from build123d import *

# Parameters (mm, degrees)
SKETCH3_R                                         = 22
BOSS_EXTRUDE1_DEPTH                               = 1.5
BOSS_EXTRUDE2_DEPTH                               = 12.5
SKETCH5_R                                         = 24.5
SKETCH5_R_2                                       = 22
BOSS_EXTRUDE3_DEPTH                               = 12.5
BOSS_EXTRUDE5_DEPTH                               = 2
CUT_REVOLVE1_ANGLE                                = 20
CIRPATTERN1_COUNT                                 = 12
SKETCH12_R                                        = 3.75
BOSS_EXTRUDE6_DEPTH                               = 5
CSK_FOR_4_FLAT_HEAD_MACHINE_SCREW_100_D           = 3.2639
CSK_FOR_4_FLAT_HEAD_MACHINE_SCREW_100_CSINK_D     = 5.715
CSK_FOR_4_FLAT_HEAD_MACHINE_SCREW_100_CSINK_ANGLE = 100


# Read off the part's stored shape, not the designer's step: Cut-Revolve1
with BuildPart() as part:
    # Sketch3 → Boss-Extrude1 (new body)
    with BuildSketch(Plane(origin=(0, 0, 0), x_dir=(1, 0, 0), z_dir=(0, 1, 0))):
        with BuildLine():
            Line((39.523027355, 46), (34.965412665, 46))
            Line((34.965412665, 46), (-7.331355166, 37.795518669))
            ThreePointArc((-7.331355166, 37.795518669), (-22.480334206, 31.255152759), (-33.5, 18.973665961))
            Line((-33.5, 18.973665961), (-33.5, -18.973665961))
            ThreePointArc((-33.5, -18.973665961), (-3.369315914, -38.35228429), (29.67865128, -24.524022064))
            Line((29.67865128, -24.524022064), (58.016889207, 9.770543449))
            ThreePointArc((58.016889207, 9.770543449), (58.612248226, 10.815349677), (58.81883, 12))
            Line((58.81883, 12), (58.81883, 32.5))
            ThreePointArc((58.81883, 32.5), (58.362392683, 34.228214743), (57.112129316, 35.505674228))
            Line((57.112129316, 35.505674228), (39.523027355, 46))
        make_face()
        with Locations(Location((0, 0, 0), (0, 0, 270))):
            Circle(SKETCH3_R, mode=Mode.SUBTRACT)
    extrude(amount=BOSS_EXTRUDE1_DEPTH)

    # Sketch4 → Boss-Extrude2 (add)
    with BuildSketch(Plane(origin=(0, 1.5, 0), x_dir=(1, 0, 0), z_dir=(0, 1, 0))):
        with BuildLine():
            Line((57.112129316, 35.505674228), (39.523027355, 46))
            Line((39.523027355, 46), (34.965412665, 46))
            Line((34.965412665, 46), (-7.331355166, 37.795518669))
            ThreePointArc((-7.331355166, 37.795518669), (-22.480334206, 31.255152759), (-33.5, 18.973665961))
            Line((-33.5, 18.973665961), (-33.5, -18.973665961))
            ThreePointArc((-33.5, -18.973665961), (-3.369315914, -38.35228429), (29.67865128, -24.524022064))
            Line((29.67865128, -24.524022064), (58.016889207, 9.770543449))
            ThreePointArc((58.016889207, 9.770543449), (58.612248226, 10.815349677), (58.81883, 12))
            Line((58.81883, 12), (58.81883, 32.5))
            ThreePointArc((58.81883, 32.5), (58.362392683, 34.228214743), (57.112129316, 35.505674228))
        make_face()
        with BuildLine():
            Line((55.831201233, 33.358764065), (38.83389843, 43.5))
            Line((38.83389843, 43.5), (35.205641557, 43.5))
            Line((35.205641557, 43.5), (-6.855293142, 35.34126421))
            ThreePointArc((-6.855293142, 35.34126421), (-20.756477834, 29.413748961), (-31, 18.303005218))
            Line((-31, 18.303005218), (-31, -18.303005218))
            ThreePointArc((-31, -18.303005218), (-2.827385178, -35.888798992), (27.751466132, -22.931553099))
            Line((27.751466132, -22.931553099), (56.089704059, 11.363012414))
            ThreePointArc((56.089704059, 11.363012414), (56.259806636, 11.661528479), (56.31883, 12))
            Line((56.31883, 12), (56.31883, 32.5))
            ThreePointArc((56.31883, 32.5), (56.188419338, 32.993775641), (55.831201233, 33.358764065))
        make_face(mode=Mode.SUBTRACT)
    extrude(amount=BOSS_EXTRUDE2_DEPTH)

    # Sketch5 → Boss-Extrude3 (add)
    with BuildSketch(Plane(origin=(0, 1.5, 0), x_dir=(1, 0, 0), z_dir=(0, 1, 0))):
        with Locations(Location((0, 0, 0), (0, 0, 270))):
            Circle(SKETCH5_R)
        with Locations(Location((0, 0, 0), (0, 0, 270))):
            Circle(SKETCH5_R_2, mode=Mode.SUBTRACT)
    extrude(amount=BOSS_EXTRUDE3_DEPTH)

    # Sketch8 → Boss-Extrude5 (add)
    with BuildSketch(Plane(origin=(0, 14, 0), x_dir=(1, 0, 0), z_dir=(0, 1, 0))):
        with BuildLine():
            Line((57.112129316, 35.505674228), (39.523027355, 46))
            Line((39.523027355, 46), (34.965412665, 46))
            Line((34.965412665, 46), (-7.331355166, 37.795518669))
            ThreePointArc((-7.331355166, 37.795518669), (-22.480334206, 31.255152759), (-33.5, 18.973665961))
            Line((-33.5, 18.973665961), (-33.5, -18.973665961))
            ThreePointArc((-33.5, -18.973665961), (-3.369315914, -38.35228429), (29.67865128, -24.524022064))
            Line((29.67865128, -24.524022064), (58.016889207, 9.770543449))
            ThreePointArc((58.016889207, 9.770543449), (58.612248226, 10.815349677), (58.81883, 12))
            Line((58.81883, 12), (58.81883, 32.5))
            ThreePointArc((58.81883, 32.5), (58.362392683, 34.228214743), (57.112129316, 35.505674228))
        make_face()
        with BuildLine():
            Line((35.061504222, 45), (-7.140930356, 36.813816885))
            ThreePointArc((-7.140930356, 36.813816885), (-21.78998379, 30.519610194), (-32.5, 18.708286934))
            Line((-32.5, 18.708286934), (-32.5, -18.708286934))
            ThreePointArc((-32.5, -18.708286934), (-3.151328713, -37.367353764), (28.907777221, -23.887034478))
            Line((28.907777221, -23.887034478), (57.246015148, 10.407531035))
            ThreePointArc((57.246015148, 10.407531035), (57.67127159, 11.153821198), (57.81883, 12))
            Line((57.81883, 12), (57.81883, 32.5))
            ThreePointArc((57.81883, 32.5), (57.492803345, 33.734439102), (56.599758083, 34.646910163))
            Line((56.599758083, 34.646910163), (39.247375785, 45))
            Line((39.247375785, 45), (35.061504222, 45))
        make_face(mode=Mode.SUBTRACT)
    extrude(amount=BOSS_EXTRUDE5_DEPTH)

    # Cut-Revolve1 outline → Cut-Revolve1 (revolve, cut)
    with BuildSketch(Plane(origin=(0, 0, 0), x_dir=(0.984807753012208, 0, 0.17364817766693078), z_dir=(-0.17364817766693078, 0, 0.984807753012208))):
        Polygon((22, 2), (22, 0), (24.5, 2.5), (24.5, 4.5), align=None)
    cut_revolve1 = revolve(axis=Axis((0, 0, 0), (0, 1, 0)), revolution_arc=CUT_REVOLVE1_ANGLE, mode=Mode.SUBTRACT)

    # CirPattern1: Cut-Revolve1 ×12 about axis
    cirpattern1_axis = Axis((0, 0, 0), (0, 1, 0))
    for i in range(1, CIRPATTERN1_COUNT):
        add(cut_revolve1.rotate(cirpattern1_axis, i * 360 / CIRPATTERN1_COUNT), mode=Mode.SUBTRACT)

    # Sketch12 → Boss-Extrude6 (add)
    with BuildSketch(Plane(origin=(0, 0, 0), x_dir=(1, 0, 0), z_dir=(0, 1, 0))):
        with Locations((-24.04163056, 24.04163056)):
            Circle(SKETCH12_R)
        with Locations((-24.04163056, -24.04163056)):
            Circle(SKETCH12_R)
        with Locations((24.04163056, -24.04163056)):
            Circle(SKETCH12_R)
        with Locations((47.21419, 3.761759805)):
            Circle(SKETCH12_R)
        with Locations((35.10955, 41.444082154)):
            Circle(SKETCH12_R)
    extrude(amount=BOSS_EXTRUDE6_DEPTH)

    # CSK for #4 Flat Head Machine Screw (100)1 (through all)
    with Locations(Plane(origin=(0, 0, 0), x_dir=(-1, 0, 0), z_dir=(0, -1, 0))):
        with Locations((-35.10955, 41.444082154), (-47.21419, 3.761759805), (-24.04163056, -24.04163056), (24.04163056, -24.04163056), (24.04163056, 24.04163056)):
            CounterSinkHole(CSK_FOR_4_FLAT_HEAD_MACHINE_SCREW_100_D / 2, CSK_FOR_4_FLAT_HEAD_MACHINE_SCREW_100_CSINK_D / 2, counter_sink_angle=CSK_FOR_4_FLAT_HEAD_MACHINE_SCREW_100_CSINK_ANGLE)


solid = part.part
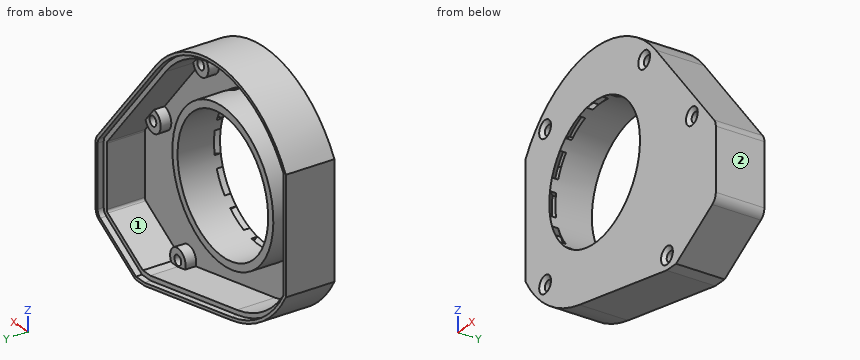
Source: CAD feature listing. Evaluate the final solid. Frame: model axes, mm. Face numbers are marked on the shaded views. A direction names the side the tool comes from. Give positions to 0.01 mm unless a question says otherwise; leave off trailing zeros. Order: outer loops, then holes, each group sorted by start corner. A loop starts at its lowest first (then second) coordinate and runs counter-clockwise, first axis right, second up. Notation, with made-up numbers: (-3.5, -31.75) -> (43.5, -31.75) arc R22 cw to (43.5, 6.25) -> close; hole circle Ø10 at (82, 41.5). An arc over 180 degrees is marked (long way). Write item = value, one per line.
Item 1: Contact query for flat-ended pins moving along their axis: pin 1 (1.6 mm diameter, centred on y = 14.5, z = 5.5, fed in from +X); pin 2 (4 mm diameter, centred on x = 37, y = 6.5, fed in from +Z); pin 3 (0.6 mm diameter, centred on x = 37, y = 15, fed in from +Z). Output: stop coordinate, or through.
Check result:
pin_1 = 46.06
pin_2 = 18.08
pin_3 = 16.03
Item 2: Set-up query: the marked faces 1 and 2. Return all of +Z, -Z, +X, -X, +Y, -Y with unobstructed straight access to the full face (end or side cutting, diameter ignored); none if empty.
Check result:
face_1 = +Y
face_2 = +Z, -Z, +X, +Y, -Y
Item 3: Section query B-B (x = 0). Output: boundary loops of the cut face in (y, z), then the cut area to 3 significant figures.
Check result:
outline = (0, -39.22) -> (16, -39.22) -> (16, -38.2) -> (14, -38.2) -> (14, -36.67) -> (1.5, -36.67) -> (1.5, -24.5) -> (2.5, -24.5) -> (0, -22) -> close; (0, 22) -> (2.5, 24.5) -> (1.5, 24.5) -> (1.5, 36) -> (14, 36) -> (14, 37.5) -> (16, 37.5) -> (16, 38.5) -> (0, 38.5) -> close; (2, -22) -> (4.5, -24.5) -> (14, -24.5) -> (14, -22) -> close; (2, 22) -> (14, 22) -> (14, 24.5) -> (4.5, 24.5) -> close
area = 170 mm²
Item 4: Section query A-A (y = 7.75). Output: boundary loops of the cut face in (x, z).
Check result:
outline = (-33.5, -18.97) arc R38.5 ccw to (-7.33, -37.8) -> (34.97, -46) -> (39.52, -46) -> (57.11, -35.51) arc R3.5 ccw to (58.82, -32.5) -> (58.82, -12) arc R3.5 ccw to (58.02, -9.77) -> (29.68, 24.52) arc R38.5 ccw to (-33.5, 18.97) -> close; circle Ø49 at (0, 0); hole (-31, -18.3) arc R36 ccw to (-6.86, -35.34) -> (35.21, -43.5) -> (38.83, -43.5) -> (55.83, -33.36) arc R1 ccw to (56.32, -32.5) -> (56.32, -12) arc R1 ccw to (56.09, -11.36) -> (27.75, 22.93) arc R36 ccw to (-31, 18.3) -> close; hole circle Ø44 at (0, 0)
Item 5: Ray query, probe 1 along Z at (x, y) = (4, 4.25); probe 2 along X at (y, z) = (11.25, 0); probe 3 along Z at (x, y) = (-9, 3.5). Return the intervals inside material, ascending.
Check result:
probe_1 = -39.99 to -37.45, -23.92 to -21.63, 21.63 to 23.92, 35.78 to 38.29
probe_2 = -33.5 to -31, -24.5 to -22, 22 to 24.5, 46.7 to 49.94
probe_3 = -37.43 to -34.86, -21.71 to -20.07, 20.07 to 21.71, 34.86 to 37.43
